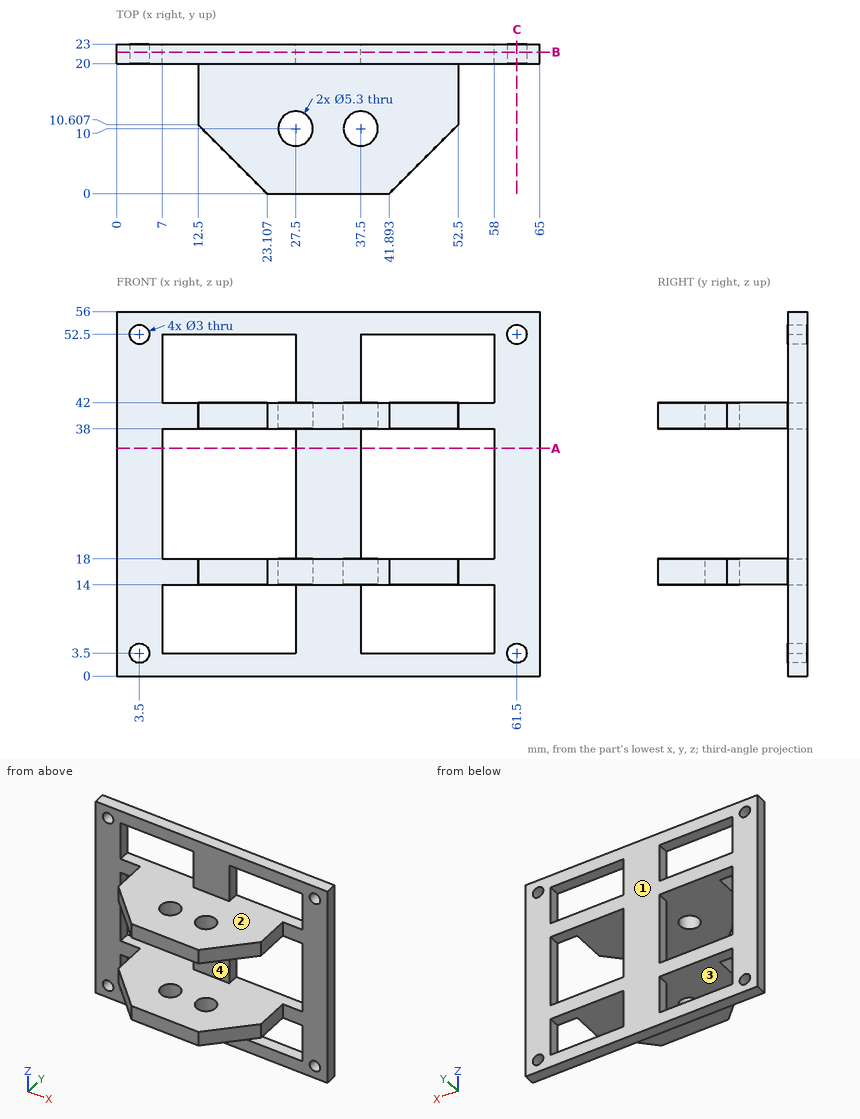
Study the drawing (mm; zero at the part's minimum x, y, z) and answer. A direction names the side the tool comes from. Coordinates: 2 decimals unless noted, no trailing zeros. Write each loop counter-clockwise with the first axis right and the second up, starting at its lowest first coordinate (ties: lowest second). Pieces come first, ordered by that corner, then holes. Notation, with made-up numbers: (1, 36) - (24, 36) arc R20 ccw to (24, 68) - close; hole circle Ø10 at (7.25, 63). An arc over 180 degrees is marked (long way). Answer as a JSON object with one key per item and string values.
Q1. Which of the six approach directions +Z, -Z, +X, -X, +Y, -Y give full straight-line access (tool end or side, diameter ignored) to the marked faces 1 and 2?
Results list:
{"face 1": "+Z, -Z, +X, -X, +Y", "face 2": "-Y"}
Q2. Consider L1, parallel to Z at x = 8.5, y = 20.25; L2, parallel to Z at x = 52, y = 13.5; L3, parallel to X at y = 19, z = 15. Determine where each line is inside the solid, lowest interval first. Write a range as from..to.
Results list:
{"L1": "z = 0..3.5, 14..18, 38..42, 52.5..56", "L2": "z = 14..18, 38..42", "L3": "x = 12.5..52.5"}
Q3. Given pin 1 Ø11.5 at (x, y) = (23.5, 17) entering from +Z; pin 2 Ø6 at (y, z) = (16, 34.5) entering from +X; pin 3 Ø3 at (y, z) = (13, 16) entering from +X; pin 4 Ø1.5 at (x, z) = (54.5, 39.5) entering from -Y, each flat-ended and moving along its own axis, determine where each tip first touches the part or whether it passes through.
Results list:
{"pin 1": "stops at z = 56", "pin 2": "passes through", "pin 3": "stops at x = 52.5", "pin 4": "stops at y = 20"}
Q4. Find section C-C (x = 61.5). Write down the section's boundary in (y, z), plus the area to 3 significant figures.
Results list:
{"outline": "(20, 0) - (23, 0) - (23, 2) - (20, 2) - close; (20, 5) - (23, 5) - (23, 51) - (20, 51) - close; (20, 54) - (23, 54) - (23, 56) - (20, 56) - close", "area": "150 mm^2"}
Q5. For a pull along X with two mould halves and no side action, classify the marked faces 3 and 4 as pulls with the +X half, pulls with the -X half, needs draft (parallel to the pull), parting line crosses it, or undercut.
Results list:
{"face 3": "undercut", "face 4": "needs draft"}
Q6. Find section B-B (y = 21.75). State how many separate pieces and enclosed holes the cut face has, plus the area to 3 significant figures.
Results list:
{"separate pieces": "1", "enclosed holes": "10", "area": "1,930 mm^2"}
Q7. Find section A-A (z = 35). Write down the section's boundary in (x, y).
Results list:
{"outline": "(0, 20) - (7, 20) - (7, 23) - (0, 23) - close; (27.5, 20) - (37.5, 20) - (37.5, 23) - (27.5, 23) - close; (58, 20) - (65, 20) - (65, 23) - (58, 23) - close"}
